Autodesk Inventor part; units mm, degrees
ref_plane "РабПлоскость1" through (0, 0, -2.75) normal (0, 0, 1) x (1, 0, 0)
ref_plane "РабПлоскость2" through (0, 0, -14.25) normal (0, 0, -1) x (-1, 0, 0)
ref_plane "YZ Plane" through (0, 0, 0) normal (1, 0, 0) x (0, 1, 0)
sketch "Эскиз6" plane through (0, 0, 0) normal (0, 0, 1) x (1, 0, 0)
  circle A0 centre (0, 0) radius 7.5
  dimension "d27" = 15
extrude "Выдавливание2" add sketch "Эскиз6" against normal blind 17
sketch "Эскиз8" plane through (0, 0, 0) normal (0, 0, 1) x (1, 0, 0)
  point P0 (0, 0)
  point P1 (0, 0)
hole "Отверстие1" at (0, 0, 0) direction (0, 0, -1) diameter 8 end through all
ref_plane "РабПлоскость1" through (0, 0, -2.75) normal (0, 0, 1) x (1, 0, 0)
ref_plane "РабПлоскость2" through (0, 0, -14.25) normal (0, 0, -1) x (-1, 0, 0)
sketch "Эскиз10" plane through (0, 0, -14.25) normal (0, 0, -1) x (-1, 0, 0)
  circle A0 centre (0, 0) radius 7.15
  circle A1 centre (0, 0) radius 7.5
  dimension "d40" = 14.3
  dimension "d41" = 15
sketch "Эскиз11" plane through (0, 0, -2.75) normal (0, 0, 1) x (1, 0, 0)
  circle A0 centre (0, 0) radius 7.15
  circle A1 centre (0, 0) radius 7.5
  dimension "d42" = 14.3
  dimension "d43" = 15
extrude "Выдавливание3" cut sketch "Эскиз11" against normal blind 1.1
extrude "Выдавливание4" cut sketch "Эскиз10" against normal blind 1.1
sketch "Эскиз12" plane through (0, 0, -17) normal (0, 0, -1) x (-1, 0, 0)
  circle A0 centre (0, 0) radius 7
  circle A1 centre (0, 0) radius 4.5
  dimension "d48" = 14
  dimension "d49" = 9
extrude "Выдавливание5" cut sketch "Эскиз12" against normal blind 0.35
sketch "Эскиз13" plane through (0, 0, 0) normal (0, 0, 1) x (1, 0, 0)
  circle A0 centre (0, 0) radius 4.5
  circle A1 centre (0, 0) radius 7
  dimension "d52" = 9
  dimension "d53" = 14
extrude "Выдавливание6" cut sketch "Эскиз13" against normal blind 0.35
chamfer "Фаска1" distance 0.35 angle 45 2 edges at (-7.5, 0, 0) (-7.5, 0, -17)
properties part number "LM8"
Geometry: final body of the model. Coordinates: model frame, mm. A direction names the side the tool comes from. Coordinates: 2 decimals unless noted, no trailing zeros. Write each loop counter-clockwise with the first axis right and the second up, starting at its lowest first coordinate (ties: lowest second). Pieces come first, ordered by that corner, then holes. Notation, with made-up numbers: (9.25, 51) - (54.25, 51) arc R20 ccw to (54.25, 89) - close; hole circle Ø10 at (31, -21). An arc over 180 degrees is marked (long way). Return JSON: item names as keys, results as strings.
Item 1: Reachability of faces 4 (the face through (0, -5, -0.35)), 5 (the face through (0.59, 4.46, -16.83)), 6 (the face through (0.93, 7.09, -13.71)) from +Z, -Z, +X, -X, +Y, -Y: full face, straight path, thin tool, end or side. Return the list, or none.
Completed:
{"face 4": "+Z", "face 5": "-Z", "face 6": "none"}
Item 2: Pin query (flat end, axial travel): pin 1 Ø5 at (x, y) = (0, 0) entering from -Z; pin 2 Ø3 at (y, z) = (5, -7.5) entering from -X; pin 3 Ø3 at (x, z) = (-3, -2.5) entering from +Y; pin 4 Ø2 at (x, z) = (-2, -12.5) entering from +Y. Return the tip coordinate at first contact, or that it passes through.
Completed:
{"pin 1": "passes through", "pin 2": "stops at x = -6.63", "pin 3": "stops at y = 7.35", "pin 4": "stops at y = 7.43"}
Item 3: Section query B-B (z = -6). Output: boundary loops of the cut face in (x, y), and give its area (3 significant figures).
Completed:
{"outline": "circle Ø15 at (0, 0); hole circle Ø8 at (0, 0)", "area": "126 mm2"}
Item 4: Pull-direction query (Z, two-part tool) for faces 1 (the face through (-0.59, 4.46, -0.17)), 2 (the face through (-0.93, 7.09, -3.29)), 3 (the face through (0, -5, -16.65)); classes: +Z half, -Z half, draft (parallel to the pull), parting line (faces both ways), or undercut.
Completed:
{"face 1": "draft", "face 2": "undercut", "face 3": "-Z half"}
Item 5: Line query: L1, parallel to Y at x = 0, z = -16.7; L2, parallel to Y at x = 0, z = -0.2; L3, parallel to Z at x = -2, y = -4.25. Output: solid intervals per line, ascending.
Completed:
{"L1": "y = -7.45 to -7, -4.5 to -4, 4 to 4.5, 7 to 7.45", "L2": "y = -7.35 to -7, -4.5 to -4, 4 to 4.5, 7 to 7.35", "L3": "z = -16.65 to -0.35"}
Item 6: Section query A-A (z = -3.5). Output: boundary loops of the cut face in (x, y), and give its area (3 significant figures).
Completed:
{"outline": "circle Ø14.3 at (0, 0); hole circle Ø8 at (0, 0)", "area": "110 mm2"}
